from build123d import *

# Parameters (mm, degrees)
F1_DEPTH    = 63.5
F2_T        = -2.54
F3_R        = 5.08
F4_T1_DEPTH = 110.49
F4_T3_DEPTH = 101.6
F4_T5_DEPTH = 110.49
F4_T7_DEPTH = 237.49
F4_T9_DEPTH = 152.4


# Not quite as in the source:
# - a fillet or chamfer that OpenCascade refuses, or shapes differently, is made with other operations: its cross-section is extruded or revolved along the edge and cut away or added


with BuildPart() as f1:
    # F0 (on Top) → F1 (new body)
    with BuildSketch(Plane.XY):
        Polygon((-32.2156401169, 127.5564689514), (-57.6156401169, 55.7144199828), (-57.6156401169, -147.4855800172), (69.3843598831, -147.4855800172), (69.3843598831, 55.7144199828), (43.9843598831, 127.5564689514), align=None)
    extrude(amount=F1_DEPTH)

    # F2
    f2_openings = [f1.faces().sort_by_distance(p)[0] for p in [
        (5.88436, -16.224771, 63.5),
    ]]
    offset(amount=F2_T, openings=f2_openings)

    # F3
    f3_edges = [f1.edges().sort_by_distance(p)[0] for p in [
        (54.516334, 90.147547, 2.54),
        (5.88436, 125.016469, 2.54),
        (-42.747615, 90.147547, 2.54),
        (-55.07564, -44.833478, 2.54),
        (5.88436, -144.94558, 2.54),
        (66.84436, -44.833478, 2.54),
    ]]
    fillet(f3_edges, radius=F3_R)

    # F4: fillet of radius 5.08 on 6 edges, made by hand

    # F4_s2 → F4_t1 (cut)
    with BuildSketch(Plane(origin=(40.7409485113, 115.2328038573, 0), x_dir=(0, 0, 1), z_dir=(-0.3333333333, -0.9428090416, 0))):
        with BuildLine():
            ThreePointArc((63.5, 67.8120197664), (62.0121024484, 71.4041222148), (58.42, 72.8920197664))
            Line((58.42, 72.8920197664), (63.5, 72.8920197664))
            Line((63.5, 72.8920197664), (63.5, 67.8120197664))
        make_face()
    extrude(amount=F4_T1_DEPTH, mode=Mode.SUBTRACT)

    # F4_s4 → F4_t3 (cut)
    with BuildSketch(Plane.YZ.offset(-44.9156401169)):
        with BuildLine():
            ThreePointArc((122.4764689514, 63.5), (126.0685713998, 62.0121024484), (127.5564689514, 58.42))
            Line((127.5564689514, 58.42), (127.5564689514, 63.5))
            Line((127.5564689514, 63.5), (122.4764689514, 63.5))
        make_face()
    extrude(amount=F4_T3_DEPTH, mode=Mode.SUBTRACT)

    # F4_s6 → F4_t5 (cut)
    with BuildSketch(Plane(origin=(-2.6033129818, 7.3632810518, 0), x_dir=(0, 0, 1), z_dir=(-0.3333333333, 0.9428090416, 0))):
        with BuildLine():
            ThreePointArc((63.5, 78.9076751698), (62.0121024484, 82.4997776182), (58.42, 83.9876751698))
            Line((58.42, 83.9876751698), (63.5, 83.9876751698))
            Line((63.5, 83.9876751698), (63.5, 78.9076751698))
        make_face()
    extrude(amount=F4_T5_DEPTH, mode=Mode.SUBTRACT)

    # F4_s8 → F4_t7 (cut)
    with BuildSketch(Plane.XZ.offset(-77.3044199828)):
        with BuildLine():
            ThreePointArc((-52.5356401169, 63.5), (-56.1277425653, 62.0121024484), (-57.6156401169, 58.42))
            Line((-57.6156401169, 58.42), (-57.6156401169, 63.5))
            Line((-57.6156401169, 63.5), (-52.5356401169, 63.5))
        make_face()
        with BuildLine():
            ThreePointArc((64.3043598831, 63.5), (67.8964623315, 62.0121024484), (69.3843598831, 58.42))
            Line((69.3843598831, 58.42), (69.3843598831, 63.5))
            Line((69.3843598831, 63.5), (64.3043598831, 63.5))
        make_face()
    extrude(amount=F4_T7_DEPTH, mode=Mode.SUBTRACT)

    # F4_s10 → F4_t9 (cut)
    with BuildSketch(Plane.YZ.offset(-70.3156401169)):
        with BuildLine():
            ThreePointArc((-142.4055800172, 63.5), (-145.9976824656, 62.0121024484), (-147.4855800172, 58.42))
            Line((-147.4855800172, 58.42), (-147.4855800172, 63.5))
            Line((-147.4855800172, 63.5), (-142.4055800172, 63.5))
        make_face()
    extrude(amount=F4_T9_DEPTH, mode=Mode.SUBTRACT)


solid = f1.part
Can you work these out from the model? Positions are in its coordinate system, mm. A direction names the side the tool comes from. Coordinates: 2 decimals unless noted, no trailing zeros. Write each loop counter-clockwise with the first axis right and the second up, starting at its lowest first coordinate (ties: lowest second). Pieces come first, ordered by that corner, then holes. Notation, with made-up numbers: (56, 0) -> (63, 0) arc R23 cw to (63, 24) -> close; hole circle Ø6 at (-32, -35.75). An arc over 180 degrees is marked (long way). Write each question's results on one line, items separated by ' | '. Start each with the question number.
Item 1: If we section it at B-B, the plane x = 31.5: Write out the boundary of the cut face in (y, z).
Item 2: Thinking about a two-plate mould opening in X: for faces 1 (the flat face through (6, 125.016, 35)), 2 (the cylindrical face through (56.2, 90.9, 61)), 3 (the flat face through (54.69, 89.66, 34.83)), 4 (the flat face through (6, 127.556, 29)), which applies, released by +X, released by -X, zero draft, split by the parting line, or undercut?
Item 3: I'm going to push flat-ended pins straight in: P1, Ø2, axis at x = -32.5, z = 28, coming from the +Y side; P2, Ø5, axis at y = 69, z = 47, coming from the -X side. Where does each tip first touch, or does it pass through?
Item 4: Please list where these lines run through material, in increasing order: probe 1 along Y at (x, z) = (-15.5, 37); probe 2 along X at (y, z) = (-67, 31); probe 3 along Z at (x, y) = (-26.5, 60.5).
Item 5: On a 3-axis mill with a long thin cutter (end or side, diameter ignored), from which of +Z, -Z, +X, -X, +Y, -Y can I reach the whole of each face in a straight line? I mean faces 5 (the cylindrical face through (-44.08, 91.91, 60.99)), 6 (the flat face through (-55.076, -43, 35)). Say none if no direction works.
Item 6: If we section it at A-A, the plane z = 40.5: Write out the boundary of the cut face in (x, y).
Item 7: If we section it at C-C, the plane y = -48.5: Write out the boundary of the cut face in (x, z).
Answer block:
1) outline: (-147.49, 0) -> (127.56, 0) -> (127.56, 58.42) arc R5.08 ccw to (125.02, 62.82) -> (125.02, 7.62) arc R5.08 cw to (119.94, 2.54) -> (-139.87, 2.54) arc R5.08 cw to (-144.95, 7.62) -> (-144.95, 62.82) arc R5.08 ccw to (-147.49, 58.42) -> close
2) face 1: undercut | face 2: released by +X | face 3: undercut | face 4: zero draft
3) P1: y = 127.56 | P2: x = -53.8
4) probe 1: -147.49 to -144.95, 125.02 to 127.56 | probe 2: -57.62 to -55.08, 66.84 to 69.38 | probe 3: 0 to 2.54
5) face 5: +Z, -X, +Y | face 6: +Z
6) outline: (-57.62, -147.49) -> (69.38, -147.49) -> (69.38, 55.71) -> (43.98, 127.56) -> (-32.22, 127.56) -> (-57.62, 55.71) -> close; hole (-55.08, -144.95) -> (66.84, -144.95) -> (66.84, 55.28) -> (42.19, 125.02) -> (-30.42, 125.02) -> (-55.08, 55.28) -> close
7) outline: (-57.62, 0) -> (69.38, 0) -> (69.38, 58.42) arc R5.08 ccw to (66.84, 62.82) -> (66.84, 7.62) arc R5.08 cw to (61.76, 2.54) -> (-50, 2.54) arc R5.08 cw to (-55.08, 7.62) -> (-55.08, 62.82) arc R5.08 ccw to (-57.62, 58.42) -> close
